Here's how the part is built. I have some questions about the finished solid (model axes, mm). Coordinates: 2 decimals unless noted, no trailing zeros. Write each loop counter-clockwise with the first axis right and the second up, starting at its lowest first coordinate (ties: lowest second). Pieces come first, ordered by that corner, then holes. Notation, with made-up numbers: (87, 52.25) -> (93, 52.25) arc R10 cw to (93, 62.25) -> close; hole circle Ø9 at (-27.75, 31). An arc over 180 degrees is marked (long way). Put each result on its own line as item: value. Start each with the question number.
Item 1: I want a section at A-A, the plane z = 203.5. List the corners of the cut face in (x, y) for me, then the cut area to 3 significant figures.
Item 2: If we mould it in two halves opening along X, with no side actions, what happens to faces 1 (the face through (6, -1, 148)), 2 (the face through (0, -4, 148)), 3 (the face through (0, -0.5, 235.5))? For each: released by +X, released by -X, zero draft, split by the parting line, or undercut.
Item 3: For pin 1 (1.8 mm diameter, centred on x = -1.5, z = 213.5, fed in from +Y); pin 2 (3 mm diameter, centred on x = 0, z = 62.5, fed in from +Y), each with a flat end and sliding along its axis, tell me the tip position at first contact or that it passes through.
Item 4: I need wall thicknesses on line 1 (X direction, y = -1.9, z = 287.5); line 2 (X direction, y = 3.5, z = 212); line 3 (Y direction, x = -5.5, z = 19). Which ranges of each line are inside material? Lowest first, please. Write a range as [from, to].
from build123d import *

# Parameters (mm, degrees)
BOSS_EXTRUDE1_DEPTH = 300
CHAMFER1_SIZE       = 0.3
LPATTERN1_COUNT     = 12
LPATTERN1_PITCH     = 25


with BuildPart() as part:
    # Sketch1 → Boss-Extrude1 (new body)
    with BuildSketch(Plane.XY):
        with BuildLine():
            Line((-6, 4), (6, 4))
            Line((6, 4), (6, 2.75))
            Line((6, 2.75), (6, 2.559016994))
            ThreePointArc((6, 2.559016994), (5.706107374, 2.475528258), (5.5, 2.25))
            Line((5.5, 2.25), (5, 2.25))
            Line((5, 2.25), (5, 1.75))
            Line((5, 1.75), (5.5, 1.75))
            ThreePointArc((5.5, 1.75), (5.706107374, 1.524471742), (6, 1.440983006))
            Line((6, 1.440983006), (6, 1.25))
            Line((6, 1.25), (6, -4))
            Line((6, -4), (-6, -4))
            Line((-6, -4), (-6, 1.25))
            Line((-6, 1.25), (-6, 1.440983006))
            ThreePointArc((-6, 1.440983006), (-5.706107374, 1.524471742), (-5.5, 1.75))
            Line((-5.5, 1.75), (-5, 1.75))
            Line((-5, 1.75), (-5, 2.25))
            Line((-5, 2.25), (-5.5, 2.25))
            ThreePointArc((-5.5, 2.25), (-5.706107374, 2.475528258), (-6, 2.559016994))
            Line((-6, 2.559016994), (-6, 2.75))
            Line((-6, 2.75), (-6, 4))
        make_face()
    extrude(amount=BOSS_EXTRUDE1_DEPTH)

    # Chamfer1
    chamfer1_edges = [part.edges().sort_by_distance(p)[0] for p in [
        (-6, 4, 150),
        (6, 4, 150),
        (6, -4, 150),
        (-6, -4, 150),
    ]]
    chamfer(chamfer1_edges, length=CHAMFER1_SIZE)

    # Sketch3 → M3 六角承窩頭蓋螺釘的柱孔1 (revolve, cut)
    with BuildSketch(Plane(origin=(0, 4, 12.5), x_dir=(0, 0, 1), z_dir=(1, 0, 0))):
        Polygon((0, 0), (0, 8), (2, 8), (1.75, 7.75), (1.75, 4.5), (3, 4.5), (3, 0.5), (3.5, 0), align=None)
    hole_wizard_m3_1 = revolve(axis=Axis((0, 10.35, 12.5), (0, -1, 0)), mode=Mode.SUBTRACT)

    # LPattern1: M3 六角承窩頭蓋螺釘的柱孔1 ×12
    with Locations(*[(0, 0, i * LPATTERN1_PITCH) for i in range(1, LPATTERN1_COUNT)]):
        add(hole_wizard_m3_1, mode=Mode.SUBTRACT)


solid = part.part
Calculated:
1. outline: (-6, -3.7) -> (-5.7, -4) -> (5.7, -4) -> (6, -3.7) -> (6, 1.44) arc R0.56 cw to (5.5, 1.75) -> (5, 1.75) -> (5, 2.25) -> (5.5, 2.25) arc R0.56 cw to (6, 2.56) -> (6, 3.7) -> (5.7, 4) -> (-5.7, 4) -> (-6, 3.7) -> (-6, 2.56) arc R0.56 cw to (-5.5, 2.25) -> (-5, 2.25) -> (-5, 1.75) -> (-5.5, 1.75) arc R0.56 cw to (-6, 1.44) -> close
1. area: 94.4 mm2
2. face 1: released by +X
2. face 2: zero draft
2. face 3: undercut
3. pin 1: stops at y = -0.5
3. pin 2: passes through
4. line 1: x = [-6, -1.75], [1.75, 6]
4. line 2: x = [-6, -2.96], [2.96, 6]
4. line 3: y = [-4, 1.75], [2.25, 4]
